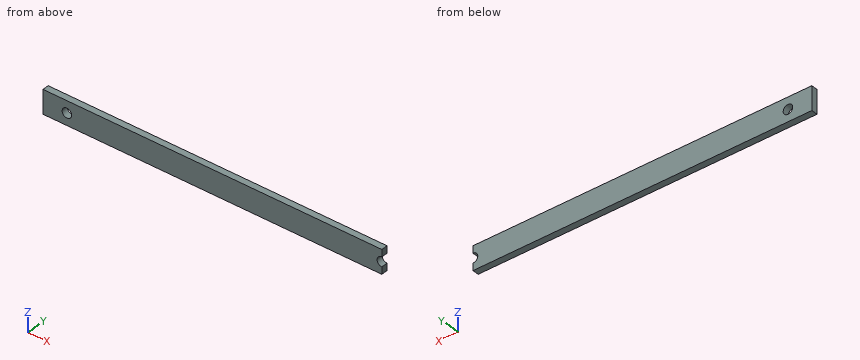
```python
from build123d import *

# Parameters (mm, degrees)
SKETCH1_W           = 212.750000014
SKETCH1_H           = 15
BOSS_EXTRUDE1_DEPTH = 4
SKETCH2_R           = 3
CUT_EXTRUDE1_DEPTH  = 107.714060116


with BuildPart() as part:
    # Sketch1 → Boss-Extrude1 (new body)
    with BuildSketch(Plane(origin=(0, 0, 0), x_dir=(1, 0, 0), z_dir=(0, 1, 0))):
        Rectangle(SKETCH1_W, SKETCH1_H)
    extrude(amount=BOSS_EXTRUDE1_DEPTH)

    # Sketch2 → Cut-Extrude1 (cut, through all)
    with BuildSketch(Plane(origin=(0, 4, 0), x_dir=(1, 0, 0), z_dir=(0, 1, 0))):
        with Locations(Location((-91.375000007, 0, 0), (0, 0, 270))):
            Circle(SKETCH2_R)
        with Locations((106.375000007, 0)):
            Circle(SKETCH2_R)
    extrude(amount=-CUT_EXTRUDE1_DEPTH, mode=Mode.SUBTRACT)


solid = part.part
```
Build history of the part. All positions in model axes, mm. Coordinates: 2 decimals unless noted, no trailing zeros. Order: outer loops, then holes, each group sorted by start corner. A loop starts at its lowest first (then second) coordinate and runs counter-clockwise, first axis right, second up.
Item 1: Drop flat-ended pins along their axis: pin 1 Ø5 at (x, z) = (70, 1.5) entering from -Y; pin 2 Ø2 at (y, z) = (2.5, -1.5) entering from +X. Give the stop position or say it passes through.
Filled in:
pin 1: stops at y = 0
pin 2: stops at x = 104.72
Item 2: Drill centre lines: L1, parallel to X at y = 0.9, z = 0 (3 decimals); L2, parallel to X at y = 0.8, z = 1.75 (3 decimals). Where is each one in solid material? Low to high.
Filled in:
L1: x = -106.375 to -94.375, -88.375 to 103.375
L2: x = -106.375 to -93.812, -88.938 to 103.938
Item 3: Saw through at A-A on z = 0. List the corners of the cut face in (x, y) (3 decimals).
Filled in:
outline: (-106.375, 0) - (-94.375, 0) - (-94.375, 4) - (-106.375, 4) - close; (-88.375, 0) - (103.375, 0) - (103.375, 4) - (-88.375, 4) - close
